Input: part model. Units: mm. Frame: model coordinates. A direction names the side the tool comes from. Round coordinates to 2 decimals unless told otherwise and drop trailing zeros. Loops run counter-clockwise (first coordinate to the right, second up) from the corner with the lowest first, then second, coordinate; pieces in that order, holes last.
1) Draft query along Y for faces 1 (the face through (16.02, 7.56, -0.98)), 2 (the face through (-2.5, 0.8, 8.6)), 3 (the face through (-9, 12, -15)). Return one class per face: pulls with the +Y half, pulls with the -Y half, needs draft (parallel to the pull), parting line crosses it, or undercut.
2) Access query for faces 4 (the face through (-7.164, 7.563, 14.368)), 5 (the face through (-8.697, 0.802, 2.136)), 6 (the face through (-8.861, 7.563, -13.388)). Directions: +Z, -Z, +X, -X, +Y, -Y. A direction counts if a zero-diameter tool reaches every point of the face in a straight line with its end or side. Return the directions, or none.
3) Ray query, line 1 along Y through (x, z) = (-8, 10.5); line 2 along Y through (x, z) = (4.5, -0.5); line 3 along Y through (x, z) = (4, -9.5). Return the intervals inside material, ascending.
4) Section C-C, the plane y = 2. Return loops of the section in (x, z).
5) First-contact query: pin 1 (5 mm diameter, centred on x = 0, z = 0, fed in from -Y); pin 2 (4 mm diameter, centred on x = 12, y = 10.5, fed in from -Z); pin 3 (12 mm diameter, centred on x = -3, z = -6, fed in from +Y); pin 4 (1 mm diameter, centred on x = -1.5, y = 2, fed in from -Z). Flat tips, straight axial feed; report the tip coordinate or a pass-through.
6) Section A-A, the plane y = 8.5. Return loops of the section in (x, z).
7) Section B-B, the plane x = 4.5. State how many separate pieces and enclosed holes the cut face has, and give its area (3 significant figures).
from build123d import *

# Parameters (mm, degrees)
REVOLVE2_ANGLE      = 7
CIRPATTERN1_COUNT   = 3
BOSS_EXTRUDE1_DEPTH = 0.5
BOSS_EXTRUDE1_DRAFT = 45
SKETCH4_R           = 14.13
BOSS_EXTRUDE2_DEPTH = 2
SKETCH5_R           = 2
CUT_EXTRUDE1_DEPTH  = 2.5


with BuildPart() as part:
    # Sketch1 → Revolve1 (revolve)
    with BuildSketch(Plane.XY, mode=Mode.PRIVATE) as revolve1_sk:
        Polygon((14, 0), (14.054310345, 3), (16.054310345, 3), (16, 0), align=None)
    revolve(revolve1_sk.sketch.rotate(Axis((0, 0, 0), (0, 1, 0)), 90), axis=Axis((0, 0, 0), (0, 1, 0)))  # turned: the seam where the file's is

    # Sketch2 → Revolve2 (revolve, symmetric)
    with BuildSketch(Plane.XY) as revolve2_sk:
        Polygon((14.054310345, 3), (16, 12), (18, 12), (16.054310345, 3), align=None)
    revolve2 = revolve(axis=Axis((0, 0, 0), (0, 1, 0)), revolution_arc=REVOLVE2_ANGLE / 2)
    revolve2 = revolve2 + revolve(revolve2_sk.sketch, axis=Axis((0, 0, 0), (0, -1, 0)), revolution_arc=REVOLVE2_ANGLE / 2)

    # CirPattern1: Revolve2 ×3 about axis
    cirpattern1_axis = Axis((0, 0, 0), (0, 1, 0))
    for i in range(1, CIRPATTERN1_COUNT):
        add(revolve2.rotate(cirpattern1_axis, i * 360 / CIRPATTERN1_COUNT))



with BuildPart() as body_2:
    # Sketch3 → Boss-Extrude1 (with draft: the straight prism first)
    with BuildSketch(Plane(origin=(0, 0.5, 0), x_dir=(1, 0, 0), z_dir=(0, 1, 0))):
        with BuildLine():
            ThreePointArc((11.674359761, 0), (8.814058264, 2.414331812), (5.109549882, 2.95))
            ThreePointArc((5.109549882, 2.95), (6.497901814, 6.426032461), (5.837179881, 10.110292126))
            ThreePointArc((5.837179881, 10.110292126), (2.316156449, 8.840364273), (0, 5.9))
            ThreePointArc((0, 5.9), (-2.316156449, 8.840364273), (-5.837179881, 10.110292126))
            ThreePointArc((-5.837179881, 10.110292126), (-6.497901814, 6.426032461), (-5.109549882, 2.95))
            ThreePointArc((-5.109549882, 2.95), (-8.814058264, 2.414331812), (-11.674359761, 0))
            ThreePointArc((-11.674359761, 0), (-8.814058264, -2.414331812), (-5.109549882, -2.95))
            ThreePointArc((-5.109549882, -2.95), (-6.497901814, -6.426032461), (-5.837179881, -10.110292126))
            ThreePointArc((-5.837179881, -10.110292126), (-2.316156449, -8.840364273), (0, -5.9))
            ThreePointArc((0, -5.9), (2.316156449, -8.840364273), (5.837179881, -10.110292126))
            ThreePointArc((5.837179881, -10.110292126), (6.497901814, -6.426032461), (5.109549882, -2.95))
            ThreePointArc((5.109549882, -2.95), (8.814058264, -2.414331812), (11.674359761, 0))
        make_face()
    extrude(amount=BOSS_EXTRUDE1_DEPTH)
    # Boss-Extrude1: the draft: its side faces are tilted about the plane it starts from
    boss_extrude1_sides = [body_2.faces().sort_by_distance(p)[0] for p in [
        (6.497901814, 0.75, 6.426032461),
        (8.814058264, 0.75, 2.414331812),
        (8.814058264, 0.75, -2.414331812),
        (6.497901814, 0.75, -6.426032461),
        (2.316156449, 0.75, -8.840364273),
        (-2.316156449, 0.75, -8.840364273),
        (-6.497901814, 0.75, -6.426032461),
        (-8.814058264, 0.75, -2.414331812),
        (-8.814058264, 0.75, 2.414331812),
        (-6.497901814, 0.75, 6.426032461),
        (-2.316156449, 0.75, 8.840364273),
        (2.316156449, 0.75, 8.840364273),
    ]]
    draft(boss_extrude1_sides, Plane(origin=(0, 0.5, 0), x_dir=(1, 0, 0), z_dir=(0, 1, 0)), BOSS_EXTRUDE1_DRAFT)


with BuildPart() as part_1:
    add(part.part)

    add(body_2.part)  # Boss-Extrude2 merges body 2
    # Sketch4 → Boss-Extrude2 (add)
    with BuildSketch(Plane(origin=(0, 1, 0), x_dir=(1, 0, 0), z_dir=(0, 1, 0))):
        Circle(SKETCH4_R)
    extrude(amount=BOSS_EXTRUDE2_DEPTH)

    # Sketch5 → Cut-Extrude1 (cut)
    with BuildSketch(Plane(origin=(0, 3, 0), x_dir=(1, 0, 0), z_dir=(0, 1, 0))):
        with Locations(Location((0, 0, 0), (0, 0, 270))):  # turned: the seam where the file's is
            Circle(SKETCH5_R)
    extrude(amount=-CUT_EXTRUDE1_DEPTH, mode=Mode.SUBTRACT)


solid = part_1.part
Final values:
1. face 1: needs draft
1. face 2: undercut
1. face 3: pulls with the +Y half
2. face 4: +Z, +X, +Y
2. face 5: none
2. face 6: -X, +Y
3. line 1: y = 1 to 3
3. line 2: y = 0.5 to 3
3. line 3: y = 0.5 to 0.71, 1 to 3
4. outline: circle Ø32.07 at (0, 0); hole circle Ø4 at (0, 0)
5. pin 1: stops at y = 0.5
5. pin 2: passes through
5. pin 3: stops at y = 3
5. pin 4: stops at z = -16.01
6. outline: (-9.52, -14.38) arc R17.24 ccw to (-7.69, -15.43) - (-6.8, -13.64) arc R15.24 cw to (-8.41, -12.71) - close; (-9.52, 14.38) - (-8.41, 12.71) arc R15.24 cw to (-6.8, 13.64) - (-7.69, 15.43) arc R17.24 ccw to start; (15.21, -0.93) - (17.21, -1.05) arc R17.24 ccw to (17.21, 1.05) - (15.21, 0.93) arc R15.24 cw to start
7. separate pieces: 1
7. enclosed holes: 2
7. area: 75.2 mm2
